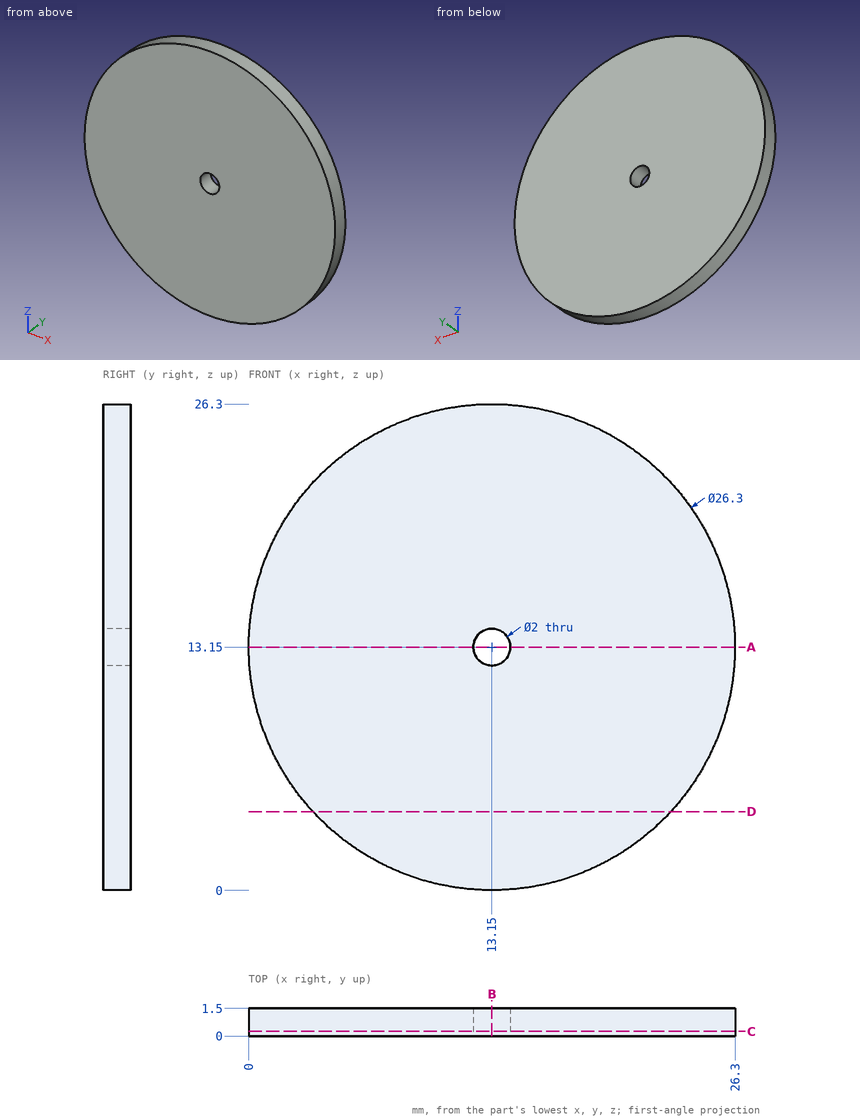
Verification items for this drawing (mm, ordinates from the low corner). Coordinates: 2 decimals unless noted, no trailing zeros. Write each loop counter-clockwise with the first axis right and the second up, starting at its lowest first coordinate (ties: lowest second). Pieces come first, ordered by that corner, then holes. Notation, with made-up numbers: M -38.5,46.5 L -8.5,46.5 A21 cw -8.5,56.5 Z; hole C 78.5,-1.75 d7. An arc over 180 degrees is marked long. Answer as a JSON object with one key per item and string values.
1. Section check C-C, the plane y = 0.25. Enter the section's corners in (x, z), plus the area to 3 significant figures.
Answers below:
{"outline": "C 13.15,13.15 d26.3; hole C 13.15,13.15 d2", "area": "540 mm²"}
2. Go/stop test with a flat-tipped pin: pin 1 Ø1.8 at (x, z) = (13.15, 13.15) entering from +Y. Record where the tip stops, or that it passes through.
Answers below:
{"pin 1": "passes through"}
3. Section check B-B, the plane x = 13.15. Enter the section's corners in (y, z), plus the area to 4 significant figures.
Answers below:
{"outline": "M 0,0 L 1.5,0 L 1.5,12.15 L 0,12.15 Z; M 0,14.15 L 1.5,14.15 L 1.5,26.3 L 0,26.3 Z", "area": "36.45 mm²"}
4. Scan lines: L1, parallel to X at y = 0.4, z = 13.15; L2, parallel to X at y = 0.5, z = 5.75; L3, parallel to Z at x = 16, y = 1.4. Record each from-to range of solid material in increasing order.
Answers below:
{"L1": "x = 0 to 12.15, 14.15 to 26.3", "L2": "x = 2.28 to 24.02", "L3": "z = 0.31 to 25.99"}
5. Section check A-A, the plane z = 13.15. Enter the section's corners in (x, y), plus the area to 4 significant figures.
Answers below:
{"outline": "M 0,0 L 12.15,0 L 12.15,1.5 L 0,1.5 Z; M 14.15,0 L 26.3,0 L 26.3,1.5 L 14.15,1.5 Z", "area": "36.45 mm²"}
6. Section check D-D, the plane z = 4.25. Enter the section's corners in (x, y).
Answers below:
{"outline": "M 3.47,0 L 22.83,0 L 22.83,1.5 L 3.47,1.5 Z"}
